Check sheet for the drawn part. Datum: minimum x, y, z corner. Units: mm. Round coordinates to 2 decimals unless told otherwise and drop trailing zeros. Write each loop counter-clockwise with the first axis right and the second up, starting at its lowest first coordinate (ties: lowest second). Pieces come first, ordered by that corner, then holes. Notation, with made-up numbers: (57.5, -15) - (104.5, -15) arc R15 cw to (104.5, -3) - close; hole circle Ø4 at (68, 17). An arc over 180 degrees is marked (long way). Answer as a JSON object with one key per item and string values.
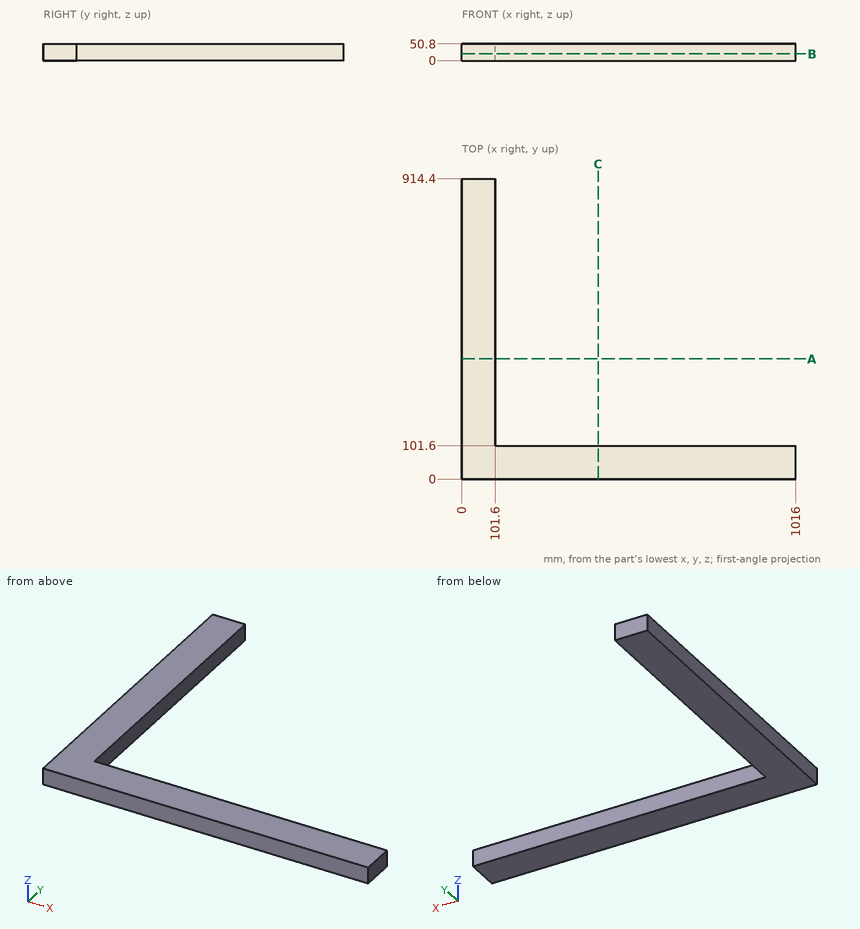
1. Material ranges on probe 1 along Y at (x, z) = (812, 47), recorded low to high. Write a range as from..to.
Completed:
{"probe 1": "y = 0..101.6"}
2. Cross-section at A-A (y = 366). Record the boundary of the cut face in (x, z).
Completed:
{"outline": "(0, 0) - (101.6, 0) - (101.6, 50.8) - (0, 50.8) - close"}
3. Go/stop test with a flat-tipped pin: pin 1 (8 mm diameter, centred on x = 679, z = 10.5, fed in from +Y). Record where the tip stops, or that it passes through.
Completed:
{"pin 1": "stops at y = 101.6"}
4. Cross-section at B-B (z = 20.5). Record the boundary of the cut face in (x, y), plus the area to 3 significant figures.
Completed:
{"outline": "(0, 0) - (1016, 0) - (1016, 101.6) - (101.6, 101.6) - (101.6, 914.4) - (0, 914.4) - close", "area": "186,000 mm^2"}
